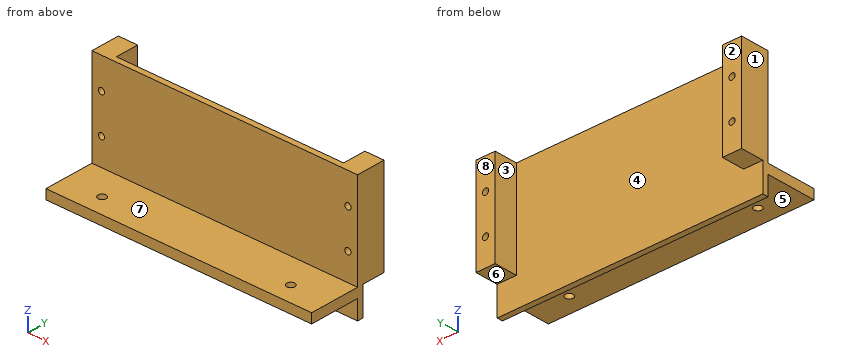
```python
from build123d import *

# Parameters (mm, degrees)
SKETCH_1_W          = 138
SKETCH_1_H          = 26
SKETCH_1_R          = 2.1
EXTRUDE_1_DEPTH     = 5
SKETCH_2_W          = 138
SKETCH_2_H          = 65
EXTRUDE_2_DEPTH     = 3
SKETCH_3_R          = 1.6
CUT_EXTRUDE_1_DEPTH = 3
SKETCH_4_W          = 10
SKETCH_4_H          = 50
SKETCH_4_R          = 1.6
EXTRUDE_3_DEPTH     = 12


with BuildPart() as part:
    # 草图1 → 凸台-拉伸1 (new body)
    with BuildSketch(Plane.XY):
        with Locations((19.202020202, 1.570004208)):
            Rectangle(SKETCH_1_W, SKETCH_1_H)
        with Locations((-29.797979798, -1.429995792)):
            Circle(SKETCH_1_R, mode=Mode.SUBTRACT)
        with Locations((68.202020202, -1.429995792)):
            Circle(SKETCH_1_R, mode=Mode.SUBTRACT)
    extrude(amount=EXTRUDE_1_DEPTH)

    # 草图2 → 凸台-拉伸2 (add)
    with BuildSketch(Plane(origin=(0, 14.570004208, 0), x_dir=(1, 0, 0), z_dir=(0, 1, 0))):
        with Locations((19.202020202, -22.5)):
            Rectangle(SKETCH_2_W, SKETCH_2_H)
    extrude(amount=EXTRUDE_2_DEPTH)

    # 草图3 → 切除-拉伸1 (cut)
    with BuildSketch(Plane(origin=(0, 17.570004208, 0), x_dir=(1, 0, 0), z_dir=(0, 1, 0))):
        with Locations((-44.797979798, -19)):
            Circle(SKETCH_3_R)
        with Locations((-44.797979798, -39)):
            Circle(SKETCH_3_R)
        with Locations((83.202020202, -19)):
            Circle(SKETCH_3_R)
        with Locations((83.202020202, -39)):
            Circle(SKETCH_3_R)
    extrude(amount=-CUT_EXTRUDE_1_DEPTH, mode=Mode.SUBTRACT)

    # 草图4 → 凸台-拉伸3 (add)
    with BuildSketch(Plane(origin=(0, 17.570004208, 0), x_dir=(1, 0, 0), z_dir=(0, 1, 0))):
        with Locations((83.202020202, -30)):
            Rectangle(SKETCH_4_W, SKETCH_4_H)
        with Locations((83.202020202, -19)):
            Circle(SKETCH_4_R, mode=Mode.SUBTRACT)
        with Locations((83.202020202, -39)):
            Circle(SKETCH_4_R, mode=Mode.SUBTRACT)
        with Locations((-44.797979798, -30)):
            Rectangle(SKETCH_4_W, SKETCH_4_H)
        with Locations((-44.797979798, -39)):
            Circle(SKETCH_4_R, mode=Mode.SUBTRACT)
        with Locations((-44.797979798, -19)):
            Circle(SKETCH_4_R, mode=Mode.SUBTRACT)
    extrude(amount=EXTRUDE_3_DEPTH)


solid = part.part
```
The listing builds one solid part. Answer for the finished solid, in the listing's coordinates (mm). Face numbers are marked on the shaded views. A direction names the side the tool comes from. Give positions to 0.01 mm unless a question says otherwise; leave off trailing zeros. Write each loop counter-clockwise with the first axis right and the second up, starting at its lowest first coordinate (ties: lowest second). Pieces come first, ordered by that corner, then holes. Notation, with made-up numbers: (23, 64) - (80, 64) arc R23 ccw to (80, 75) - close; hole circle Ø5 at (-8, -36.75). An arc over 180 degrees is marked (long way). Use one line per item in the form item = value. Start each with the question number.
1) Flat-ended cylindrical pins translate along their axes: pin 1 Ø1 at (x, y) = (29.5, 3) entering from +Z; pin 2 Ø1 at (x, z) = (71.5, -2) entering from -Y; pin 3 Ø8 at (x, y) = (-44.5, 26) entering from -Z; pin 4 Ø4 at (x, z) = (-44.8, 39) entering from +Y. Find the tip coordinate at first contact, or state that the pin passes through.
2) Find section B-B on y = 27. Determine the outline of the cut face in (x, z).
3) The mould has two halves that part along X. Classify the marked faces 1, 2, 3 and 4: pulls with the +X half, pulls with the -X half, needs draft (parallel to the pull), parting line crosses it, or undercut.
4) Find section C-C on x = 35. Determine the outline of the cut face in (y, z).
5) Find section A-A on z = 19. Determine the outline of the cut face in (x, y).
6) A tool of negligible diameter and unlimited length cuts with its end or side. For the marked faces 5, 6, 7 and 8, from which of +Z, -Z, +X, -X, +Y, -Y can it reach the whole face along a straight path? Write none if from no direction.
7) Consider line 1 along X through (y, z) = (25, 19); line 2 along X through (y, z) = (16, 19); line 3 along X through (y, z) = (27, 45.5). Determine where each line is inside the solid, lowest interval first. Write a range as from..to.
Geometry results:
q1.pin_1 = 5
q1.pin_2 = 14.57
q1.pin_3 = 5
q1.pin_4 = 29.57
q2.outline = (-49.8, 5) - (-39.8, 5) - (-39.8, 55) - (-49.8, 55) - close; (78.2, 5) - (88.2, 5) - (88.2, 55) - (78.2, 55) - close; hole circle Ø3.2 at (-44.8, 19); hole circle Ø3.2 at (-44.8, 39); hole circle Ø3.2 at (83.2, 19); hole circle Ø3.2 at (83.2, 39)
q3.face_1 = pulls with the -X half
q3.face_2 = needs draft
q3.face_3 = undercut
q3.face_4 = undercut
q4.outline = (-11.43, 0) - (14.57, 0) - (14.57, -10) - (17.57, -10) - (17.57, 55) - (14.57, 55) - (14.57, 5) - (-11.43, 5) - close
q5.outline = (-49.8, 14.57) - (-46.4, 14.57) - (-46.4, 29.57) - (-49.8, 29.57) - close; (-43.2, 14.57) - (81.6, 14.57) - (81.6, 29.57) - (78.2, 29.57) - (78.2, 17.57) - (-39.8, 17.57) - (-39.8, 29.57) - (-43.2, 29.57) - close; (84.8, 14.57) - (88.2, 14.57) - (88.2, 29.57) - (84.8, 29.57) - close
q6.face_5 = -Z, +X, -X, -Y
q6.face_6 = -Z, +X, -X, +Y
q6.face_7 = +Z, +X, -X, -Y
q6.face_8 = +Z, -Z, +X, -X, +Y
q7.line_1 = -49.8..-46.4, -43.2..-39.8, 78.2..81.6, 84.8..88.2
q7.line_2 = -49.8..-46.4, -43.2..81.6, 84.8..88.2
q7.line_3 = -49.8..-39.8, 78.2..88.2
